from build123d import *

# Parameters (mm, degrees)
SKETCH2_R             = 9
SKETCH2_R_2           = 6
LARGE_SHAFT_CUT_DEPTH = 0.5
SKETCH3_R             = 9
KEYED_SHAFT_CUT_DEPTH = 20


with BuildPart() as part:
    # Sketch2 → Large Shaft Cut (new body)
    with BuildSketch(Plane.XY):
        Circle(SKETCH2_R)
        Circle(SKETCH2_R_2, mode=Mode.SUBTRACT)
    extrude(amount=LARGE_SHAFT_CUT_DEPTH)

    # Sketch3 → Keyed Shaft Cut (add)
    with BuildSketch(Plane.XY.offset(0.5)):
        Circle(SKETCH3_R)
        with BuildLine():
            Line((-1.4, 2.765863337), (1.4, 2.765863337))
            ThreePointArc((1.4, 2.765863337), (0, -3.1), (-1.4, 2.765863337))
        make_face(mode=Mode.SUBTRACT)
    extrude(amount=KEYED_SHAFT_CUT_DEPTH)


solid = part.part
For this review, take the finished solid that the model builds, in its own axes (mm). A direction names the side the tool comes from. Coordinates: 2 decimals unless noted, no trailing zeros. Write each loop counter-clockwise with the first axis right and the second up, starting at its lowest first coordinate (ties: lowest second). Pieces come first, ordered by that corner, then holes. Notation, with made-up numbers: (-25, -34.5) -> (-8, -34.5) arc R16 cw to (-8, -26.5) -> close; hole circle Ø3 at (-22.75, 32.5). An arc over 180 degrees is marked (long way). Write each question's results on one line, items separated by ' | '. Start each with the question number.
1) Consider section C-C (z = 6.75). Write out the cut boundary in (x, y), plus the area to 3 significant figures.
2) Insertion check: pin 1 (2 mm diameter, centred on y = 3.5, z = 6, fed in from +X); pin 2 (1 mm diameter, centred on x = 4.5, z = 18, fed in from +Y); pin 3 (4 mm diameter, centred on y = -3.5, z = 13.5, fed in from -X). Each pin has a flat end and moves straight along its axis. Give the tip position at first contact, or say it passes through.
3) Consider section A-A (y = 0). Write out the cut boundary in (x, z), plus the area to 3 significant figures.
4) Consider section D-D (x = 4.5). Write out the cut boundary in (y, z), plus the area to 3 significant figures.
5) For faces 1 (the face through (0, 2.766, 10)), 2 (the face through (0, -4, 20.5)), 3 (the face through (-5.994, 0.264, 0.246)), list the 3-axis set-ups (+Z, -Z, +X, -X, +Y, -Y) from which the entire face can be reached by the end or side of a thin tool; tool diameter is ignored.
6) The part is to be moulded in two halves that separate along Y. For faces 4 (the face through (-1.172, 8.923, 10.106)), 5 (the face through (2, -6, 0)), 6 (the face through (0.1, -3.1, 10.4)), say which applies: +Y half, -Y half, draft (parallel to the pull), parting line (faces both ways), or undercut.
7) Consider section B-B (x = 0). Write out the cut boundary in (y, z), plus the area to 3 significant figures.
8) Wall thickness on L1, parallel to Y at x = 0, z = 0.35; L2, parallel to Y at x = 0, z = 19.75; L3, parallel to X at y = -1, z = 14: over which ranges is each line inside the solid? List them lowest first. Write a range as [from, to].
Geometry says:
1) outline: circle Ø18 at (0, 0); hole (-1.4, 2.77) arc R3.1 ccw (long way) to (1.4, 2.77) -> close | area: 225 mm^2
2) pin 1: x = 8.65 | pin 2: y = 8.06 | pin 3: x = -8.87
3) outline: (-9, 0) -> (-6, 0) -> (-6, 0.5) -> (-3.1, 0.5) -> (-3.1, 20.5) -> (-9, 20.5) -> close; (3.1, 0.5) -> (6, 0.5) -> (6, 0) -> (9, 0) -> (9, 20.5) -> (3.1, 20.5) -> close | area: 239 mm^2
4) outline: (-7.79, 0) -> (-3.97, 0) -> (-3.97, 0.5) -> (3.97, 0.5) -> (3.97, 0) -> (7.79, 0) -> (7.79, 20.5) -> (-7.79, 20.5) -> close | area: 316 mm^2
5) face 1: +Z, -Z | face 2: +Z, +X, -X, +Y, -Y | face 3: -Z
6) face 4: parting line | face 5: draft | face 6: undercut
7) outline: (-9, 0) -> (-6, 0) -> (-6, 0.5) -> (-3.1, 0.5) -> (-3.1, 20.5) -> (-9, 20.5) -> close; (2.77, 0.5) -> (6, 0.5) -> (6, 0) -> (9, 0) -> (9, 20.5) -> (2.77, 20.5) -> close | area: 246 mm^2
8) L1: [-9, -6], [6, 9] | L2: [-9, -3.1], [2.77, 9] | L3: [-8.94, -2.93], [2.93, 8.94]
